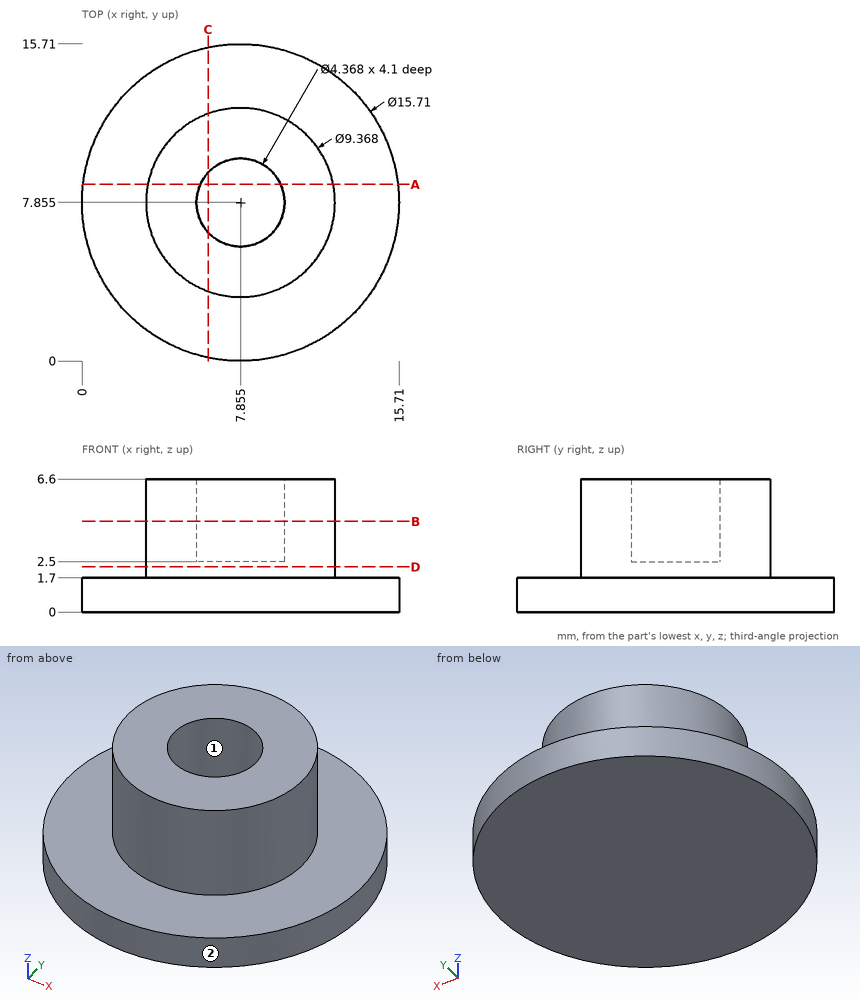
The figure shows three views and two pictorial views of one solid part (mm, origin at its lowest corner). Answer the questions. A direction names the side the tool comes from. Give positions to 0.01 mm unless a question says otherwise; leave off trailing zeros. Write each loop counter-clockwise with the first axis right and the second up, starting at its lowest first coordinate (ties: lowest second). Pieces come first, ordered by that corner, then holes. Notation, with made-up numbers: (-8, 19) - (37, 19) arc R32 cw to (37, 48) - close; hole circle Ø5 at (60.5, -36). An arc over 180 degrees is marked (long way). Return JSON: item names as keys, results as strings.
Q1. For the marked faces 1 and 2, determine the directions among +Z, -Z, +X, -X, +Y, -Y from which every point of the face is accessible in a straight line to the end or side of a thin tool.
Reply:
{"face 1": "+Z", "face 2": "+Z, -Z"}
Q2. A cutting plane is placed at C-C, the plane x = 6.25. Determine the outline of the cut face in (y, z) (1 decimal).
Reply:
{"outline": "(0.2, 0) - (15.5, 0) - (15.5, 1.7) - (12.3, 1.7) - (12.3, 6.6) - (9.3, 6.6) - (9.3, 2.5) - (6.4, 2.5) - (6.4, 6.6) - (3.5, 6.6) - (3.5, 1.7) - (0.2, 1.7) - close"}
Q3. A cutting plane is placed at A-A, the plane y = 8.75. Determine the outline of the cut face in (x, z).
Reply:
{"outline": "(0.05, 0) - (15.66, 0) - (15.66, 1.7) - (12.45, 1.7) - (12.45, 6.6) - (9.85, 6.6) - (9.85, 2.5) - (5.86, 2.5) - (5.86, 6.6) - (3.26, 6.6) - (3.26, 1.7) - (0.05, 1.7) - close"}
Q4. A cutting plane is placed at D-D, the plane z = 2.25. Determine the outline of the cut face in (x, y) (1 decimal).
Reply:
{"outline": "circle Ø9.4 at (7.9, 7.9)"}
Q5. Consider line 1 along Y through (x, z) = (7.75, 2.25); line 2 along X through (y, z) = (6, 5) (1 decimal); line 3 along Z through (x, y) = (9, 3). Determine where each line is inside the solid, lowest interval first. Write a range as [from, to].
Reply:
{"line 1": "[3.17, 12.54]", "line 2": "[3.6, 6.7], [9, 12.2]", "line 3": "[0, 1.7]"}
Q6. A cutting plane is placed at B-B, the plane z = 4.5. Determine the outline of the cut face in (x, y) (1 decimal).
Reply:
{"outline": "circle Ø9.4 at (7.9, 7.9); hole circle Ø4.4 at (7.9, 7.9)"}
Q7. Given P1, Ø3, axis at x = 4, z = 1, coming from the -Y side; P2, Ø1.5, axis at x = 5.5, z = 3, coming from the -Y side; P3, Ø1.5, axis at y = 2, z = 1.5, coming from the -X side (1 decimal), each flat-ended and moving along its own axis, determine where each tip first touches the part or whether it passes through.
Reply:
{"P1": "y = 0.36", "P2": "y = 3.45", "P3": "x = 1.9"}
